Could you check a few things on this drawing? It's one solid part, dimensions in mm from its lowest x, y, z. A direction names the side the tool comes from. Give positions to 0.01 mm unless a question says otherwise; leave off trailing zeros. Loops run counter-clockwise (first coordinate to the right, second up) from the corner with the lowest first, then second, coordinate; pieces in that order, holes last. Notation, with made-up numbers: (28, 60.25) - (35, 60.25) arc R5 cw to (35, 69.25) - close; hole circle Ø11 at (31.25, -10). An arc over 180 degrees is marked (long way). Write each question's results on one line, items separated by ' | '. Start each with the question number.
(1) Suppose I cut it at D-D (x = 3.1). Please give me the cut outline in (y, z).
(2) Suppose I cut it at C-C (y = 15.25). Please give me the cut outline in (x, z).
(3) Suppose I cut it at B-B (x = 4). Please give me the cut outline in (y, z).
(4) I need wall thicknesses on line 1 (Y direction, x = 4, z = 1.3); line 2 (Y direction, x = 0.45, z = 1.85); line 3 (X direction, y = 15.5, z = 1.8). Which ranges of each line are inside material? Lowest first, please.
(5) On a 3-axis mill with a long thin cutter (end or side, diameter ignored), from which of +Z, -Z, +X, -X, +Y, -Y can I reach the whole of each face in a straight line? I mean the marked faces 1, 2 and 3. Say none if no direction works.
(6) Suppose I cut it at A-A (z = 1.2). Please give me the cut outline in (x, y).
(7) For pin 1 (1 mm diameter, centred on y = 2.5, z = 1, fed in from +X); pin 2 (0.6 mm diameter, centred on y = 13, z = 1, fed in from -X); pin 3 (0.5 mm diameter, centred on x = 0.5, z = 0.5, fed in from -Y), each with a flat end and sliding along its axis, tell me the tip position at first contact or that it passes through.
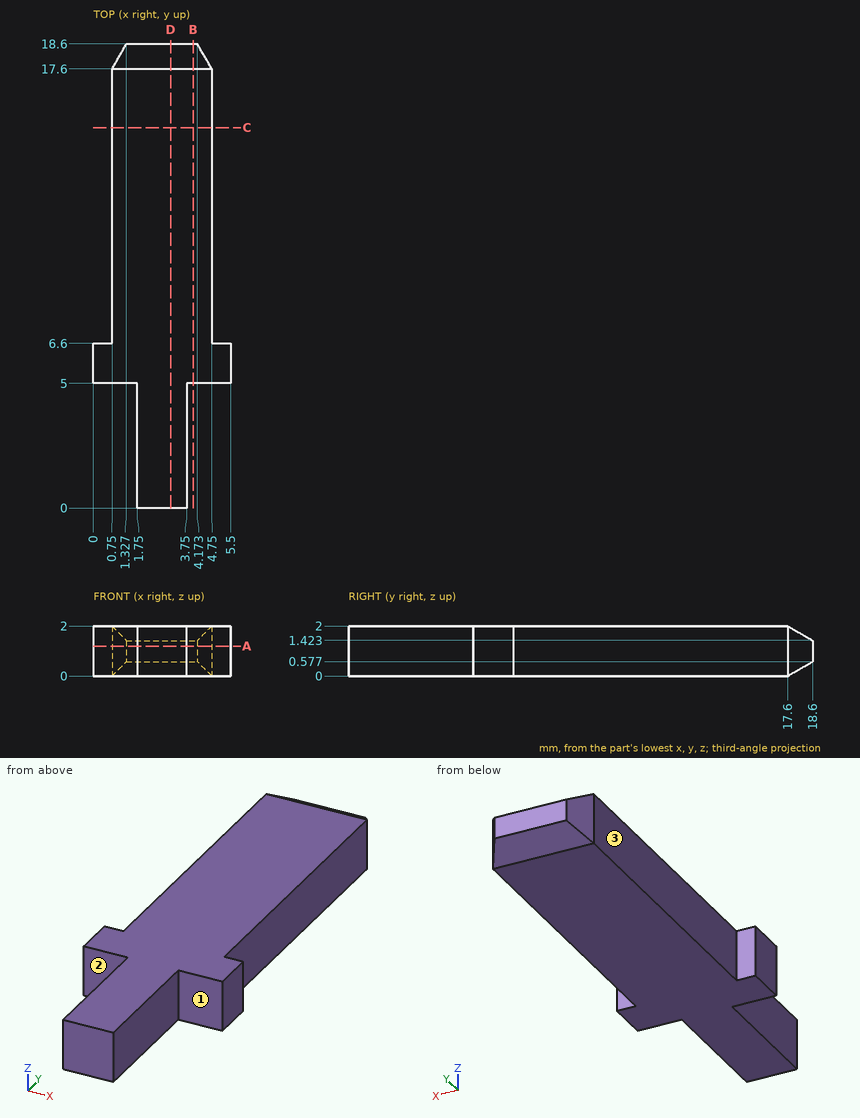
Output values:
1) outline: (0, 0) - (17.6, 0) - (18.6, 0.58) - (18.6, 1.42) - (17.6, 2) - (0, 2) - close
2) outline: (0.75, 0) - (4.75, 0) - (4.75, 2) - (0.75, 2) - close
3) outline: (5, 0) - (17.6, 0) - (18.6, 0.58) - (18.6, 1.42) - (17.6, 2) - (5, 2) - close
4) line 1: 5 to 18.6 | line 2: 5 to 6.6 | line 3: 0.75 to 4.75
5) face 1: +Z, -Z, +X, -Y | face 2: +Z, -Z, -X, -Y | face 3: +Z, -Z, -X, +Y
6) outline: (0, 5) - (1.75, 5) - (1.75, 0) - (3.75, 0) - (3.75, 5) - (5.5, 5) - (5.5, 6.6) - (4.75, 6.6) - (4.75, 17.6) - (4.17, 18.6) - (1.33, 18.6) - (0.75, 17.6) - (0.75, 6.6) - (0, 6.6) - close
7) pin 1: x = 3.75 | pin 2: x = 0.75 | pin 3: y = 5
